from build123d import *

# Parameters (mm, degrees)
SKETCH_W        = 108
SKETCH_H        = 64.4
PAD_DEPTH       = 22
SKETCH001_W     = 102
SKETCH001_H     = 58.4
POCKET_DEPTH    = 20
SKETCH002_R     = 4
PAD001_DEPTH    = 2
SKETCH003_R     = 2.4
PAD002_DEPTH    = 4
SKETCH004_R     = 4.2
SKETCH004_W     = 12
SKETCH004_H     = 1
POCKET001_DEPTH = 3
SKETCH005_W     = 12
SKETCH005_H     = 1
SKETCH005_W_2   = 14
SKETCH005_H_2   = 3
POCKET002_DEPTH = 3
SKETCH006_R     = 2.4
SKETCH006_W     = 8
SKETCH006_H     = 4
POCKET003_DEPTH = 3
SKETCH007_W     = 12
SKETCH007_H     = 2
POCKET004_DEPTH = 2
SKETCH008_W     = 12
SKETCH008_H     = 2
POCKET005_DEPTH = 2
SKETCH009_W     = 12
SKETCH009_H     = 1
POCKET006_DEPTH = 7
POCKET007_DEPTH = 1.4
POCKET008_DEPTH = 1.4
FILLET_R        = 4
FILLET001_R     = 1
CHAMFER_SIZE    = 0.6
CHAMFER001_SIZE = 1
SKETCH012_R     = 6.2
POCKET009_DEPTH = 1


with BuildPart() as part:
    # Sketch → Pad (new body)
    with BuildSketch(Plane.XY):
        Rectangle(SKETCH_W, SKETCH_H)
    extrude(amount=PAD_DEPTH)

    # Sketch001 (on Face6 of Pad) → Pocket (cut)
    with BuildSketch(Plane.XY.offset(22)):
        Rectangle(SKETCH001_W, SKETCH001_H)
    extrude(amount=-POCKET_DEPTH, mode=Mode.SUBTRACT)

    # Sketch002 (on Face11 of Pocket) → Pad001 (join)
    with BuildSketch(Plane.XY.offset(2)):
        with Locations((-43.71, 18.4)):
            Circle(SKETCH002_R)
        with Locations((45.75, 18.4)):
            Circle(SKETCH002_R)
        with Locations((45.75, -18.4)):
            Circle(SKETCH002_R)
        with Locations((-43.71, -18.4)):
            Circle(SKETCH002_R)
    extrude(amount=PAD001_DEPTH)

    # Sketch003 (on Face11 of Pad001) → Pad002 (join)
    with BuildSketch(Plane.XY.offset(2)):
        with Locations((-43.71, 18.4)):
            Circle(SKETCH003_R)
        with Locations((45.75, 18.4)):
            Circle(SKETCH003_R)
        with Locations((45.75, -18.4)):
            Circle(SKETCH003_R)
        with Locations((-43.71, -18.4)):
            Circle(SKETCH003_R)
    extrude(amount=PAD002_DEPTH)

    # Sketch004 (on Face1 of Pad002) → Pocket001 (cut)
    with BuildSketch(Plane(origin=(0, 32.2, 0), x_dir=(-1, 0, 0), z_dir=(0, 1, 0))):
        with Locations((-25.2, 9)):
            Circle(SKETCH004_R)
        with Locations((23.702, 9)):
            Circle(SKETCH004_R)
        with Locations((-36, 21.5)):
            Rectangle(SKETCH004_W, SKETCH004_H)
        with Locations((36, 21.5)):
            Rectangle(SKETCH004_W, SKETCH004_H)
    extrude(amount=-POCKET001_DEPTH, mode=Mode.SUBTRACT)

    # Sketch005 (on Face15 of Pocket001) → Pocket002 (cut)
    with BuildSketch(Plane.XZ.offset(32.2)):
        with Locations((-36, 21.5)):
            Rectangle(SKETCH005_W, SKETCH005_H)
        with Locations((36, 21.5)):
            Rectangle(SKETCH005_W, SKETCH005_H)
        with Locations((13, 5.5)):
            Rectangle(SKETCH005_W_2, SKETCH005_H_2)
    extrude(amount=-POCKET002_DEPTH, mode=Mode.SUBTRACT)

    # Sketch006 (on Face3 of Pocket002) → Pocket003 (cut)
    with BuildSketch(Plane.YZ.offset(54)):
        with Locations((-6.3, 6)):
            Circle(SKETCH006_R)
        with Locations((8.7, 6)):
            Circle(SKETCH006_R)
        with Locations((1.2, 6)):
            Rectangle(SKETCH006_W, SKETCH006_H)
    extrude(amount=-POCKET003_DEPTH, mode=Mode.SUBTRACT)

    # Sketch007 (on Face23 of Pocket003) → Pocket004 (cut)
    with BuildSketch(Plane.XZ.offset(-29.2)):
        with Locations((-36, 18)):
            Rectangle(SKETCH007_W, SKETCH007_H)
        with Locations((36, 18)):
            Rectangle(SKETCH007_W, SKETCH007_H)
    extrude(amount=-POCKET004_DEPTH, mode=Mode.SUBTRACT)

    # Sketch008 (on Face25 of Pocket004) → Pocket005 (cut)
    with BuildSketch(Plane(origin=(0, -29.2, 0), x_dir=(-1, 0, 0), z_dir=(0, 1, 0))):
        with Locations((-36, 18)):
            Rectangle(SKETCH008_W, SKETCH008_H)
        with Locations((36, 18)):
            Rectangle(SKETCH008_W, SKETCH008_H)
    extrude(amount=-POCKET005_DEPTH, mode=Mode.SUBTRACT)

    # Sketch009 (on Face31 of Pocket005) → Pocket006 (cut)
    with BuildSketch(Plane.XY.offset(22)):
        with Locations((-36, 29.7)):
            Rectangle(SKETCH009_W, SKETCH009_H)
        with Locations((36, 29.7)):
            Rectangle(SKETCH009_W, SKETCH009_H)
        with Locations((36, -29.7)):
            Rectangle(SKETCH009_W, SKETCH009_H)
        with Locations((-36, -29.7)):
            Rectangle(SKETCH009_W, SKETCH009_H)
    extrude(amount=-POCKET006_DEPTH, mode=Mode.SUBTRACT)

    # Sketch010 (on Face16 of Pocket006) → Pocket007 (cut)
    with BuildSketch(Plane.XZ.offset(32.2)):
        with BuildLine():
            ThreePointArc((6, 9), (2.5, 5.5), (6, 2))
            Line((6, 2), (20, 2))
            ThreePointArc((20, 2), (23.5, 5.5), (20, 9))
            Line((6, 9), (20, 9))
        make_face()
    extrude(amount=-POCKET007_DEPTH, mode=Mode.SUBTRACT)

    # Sketch011 (on Face3 of Pocket007) → Pocket008 (cut)
    with BuildSketch(Plane.YZ.offset(54)):
        with BuildLine():
            ThreePointArc((-5.8, 10), (-9.8, 6), (-5.8, 2))
            Line((-5.8, 2), (8.2, 2))
            ThreePointArc((8.2, 2), (12.2, 6), (8.2, 10))
            Line((-5.8, 10), (8.2, 10))
        make_face()
    extrude(amount=-POCKET008_DEPTH, mode=Mode.SUBTRACT)

    # Fillet
    fillet_edges = [part.edges().sort_by_distance(p)[0] for p in [
        (54, -32.2, 11),
        (54, 32.2, 11),
        (-54, 32.2, 11),
        (-54, -32.2, 11),
    ]]
    fillet(fillet_edges, radius=FILLET_R)

    # Fillet001
    fillet001_edges = [part.edges().sort_by_distance(p)[0] for p in [
        (-51, 29.2, 12),
        (-51, -29.2, 12),
        (51, -29.2, 12),
        (51, 29.2, 12),
    ]]
    fillet(fillet001_edges, radius=FILLET001_R)

    # Chamfer
    chamfer_edges = [part.edges().sort_by_distance(p)[0] for p in [
        (52.6, 1.2, 8),
        (52.6, -2.8, 6),
        (52.6, 5.2, 6),
        (52.6, 1.2, 4),
    ]]
    chamfer(chamfer_edges, length=CHAMFER_SIZE)

    # Chamfer001
    chamfer001_edges = [part.edges().sort_by_distance(p)[0] for p in [
        (13, -30.8, 7),
        (6, -30.8, 5.5),
        (13, -30.8, 4),
        (20, -30.8, 5.5),
    ]]
    chamfer(chamfer001_edges, length=CHAMFER001_SIZE)

    # Sketch012 (on Face43 of Chamfer001) → Pocket009 (cut)
    with BuildSketch(Plane.XZ.offset(-29.2)):
        with Locations((-23.702, 9)):
            Circle(SKETCH012_R)
        with Locations((25.2, 9)):
            Circle(SKETCH012_R)
    extrude(amount=-POCKET009_DEPTH, mode=Mode.SUBTRACT)


solid = part.part
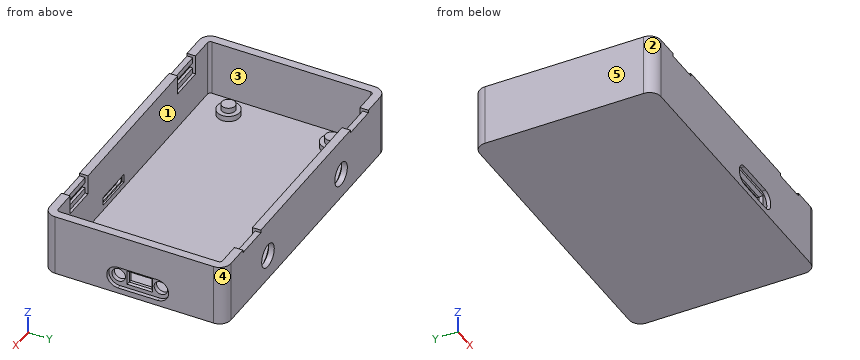
Model file for the job. Use its own axes, mm. Face numbers are marked on the shaded views. A direction names the side the tool comes from. Give positions to 0.01 mm unless a question says otherwise; leave off trailing zeros. Order: outer loops, then holes, each group sorted by start corner. A loop starts at its lowest first (then second) coordinate and runs counter-clockwise, first axis right, second up. Notation, with made-up numbers: (6.5, 14.25) -> (44.5, 14.25) arc R12 cw to (44.5, 19.25) -> close; hole circle Ø11 at (82.5, 54.5). An arc over 180 degrees is marked (long way). Use CSV: the item, a comma, the result in double quotes.
1. Band-saw the part on A-A, the plane y = 3.5. Give the cut face in (x, z).
Outcome:
outline,"(-54, 0) -> (54, 0) -> (54, 2) -> (52.6, 2) -> (52.6, 3.4) -> (52, 4) -> (51, 4) -> (51, 2) -> (-51, 2) -> (-51, 22) -> (-54, 22) -> close; (51, 8) -> (52, 8) -> (52.6, 8.6) -> (52.6, 10) -> (54, 10) -> (54, 22) -> (51, 22) -> close"
2. Mould opens along Y. For the marked faces 3, 4 and 5 say: +Y half, -Y half, draft (parallel to the pull), parting line (faces both ways), or undercut.
Outcome:
face 3,"undercut"
face 4,"+Y half"
face 5,"draft"
3. Drop flat-ended pins along their axis: pin 1 (1.1 mm diameter, centred on x = 51.5, z = 5.5, fed in from +Y); pin 2 (4 mm diameter, centred on x = -13.5, y = 24, fed in from +Z); pin 3 (0.8 mm diameter, centred on x = 51.5, z = 6.5, fed in from -Y). Give the stop position or say it passes through.
Outcome:
pin 1,"y = 32.09"
pin 2,"z = 2"
pin 3,"y = -32.05"
4. Band-saw the part on D-D, the plane y = -18.4. Give the cut face in (x, z), then the cut area to 3 significant figures.
Outcome:
outline,"(-54, 0) -> (54, 0) -> (54, 22) -> (51, 22) -> (51, 2) -> (49.75, 2) -> (49.75, 4) -> (48.15, 4) -> (48.15, 6) -> (43.35, 6) -> (43.35, 4) -> (41.75, 4) -> (41.75, 2) -> (-39.71, 2) -> (-39.71, 4) -> (-41.31, 4) -> (-41.31, 6) -> (-46.11, 6) -> (-46.11, 4) -> (-47.71, 4) -> (-47.71, 2) -> (-51, 2) -> (-51, 22) -> (-54, 22) -> close"
area,"387 mm²"
5. Band-saw the part on B-B, the plane x = 25.2. Give the cut face in (y, z), then the cut area to 3 significant figures.
Outcome:
outline,"(-32.2, 0) -> (32.2, 0) -> (32.2, 4.8) -> (30.2, 4.8) -> (30.2, 2.8) -> (29.2, 2.8) -> (29.2, 2) -> (-29.2, 2) -> (-29.2, 22) -> (-32.2, 22) -> close; (29.2, 15.2) -> (30.2, 15.2) -> (30.2, 13.2) -> (32.2, 13.2) -> (32.2, 22) -> (29.2, 22) -> close"
area,"220 mm²"
6. Drill centre lines: line 1 along X through (y, z) = (-10, 4.75); line 2 along Y through (x, z) = (-43, 10.75); line 3 along X through (y, z) = (0.5, 9.5). Where is each one in solid material? Low to high. Write a range as from..to.
Outcome:
line 1,"-54..-51, 51..54"
line 2,"-32.2..-29.2, 29.2..32.2"
line 3,"-54..-51, 51..52.6"
7. Band-saw the part on C-C, the plane x = 45.75. Give the cut face in (y, z), then the cut area to 3 significant figures.
Outcome:
outline,"(-32.2, 0) -> (32.2, 0) -> (32.2, 22) -> (29.2, 22) -> (29.2, 2) -> (22.4, 2) -> (22.4, 4) -> (20.8, 4) -> (20.8, 6) -> (16, 6) -> (16, 4) -> (14.4, 4) -> (14.4, 2) -> (-14.4, 2) -> (-14.4, 4) -> (-16, 4) -> (-16, 6) -> (-20.8, 6) -> (-20.8, 4) -> (-22.4, 4) -> (-22.4, 2) -> (-29.2, 2) -> (-29.2, 22) -> (-32.2, 22) -> close"
area,"300 mm²"
8. 3-axis set-ups, long thin cutter, end or side, ignore diameter. For the marked faces 1 and 2: which of +Z, -Z, +X, -X, +Y, -Y reach the whole face in a straight line?
Outcome:
face 1,"+Z"
face 2,"+Z, -Z, -X, -Y"
